Source: CAD feature listing. Evaluate the final solid. Frame: model axes, mm. Face numbers are marked on the shaded views. A direction names the side the tool comes from. Give positions to 0.01 mm unless a question says otherwise; leave off trailing zeros. Loops run counter-clockwise (first coordinate to the right, second up) from the corner with the lowest first, then second, coordinate; pieces in that order, holes last. Notation, with made-up numbers: M -9,14.25 L 13,14.25 A25 ccw 13,35.25 Z; hole C 11,-26 d5. An arc over 180 degrees is marked long. Write item = value, one per line.
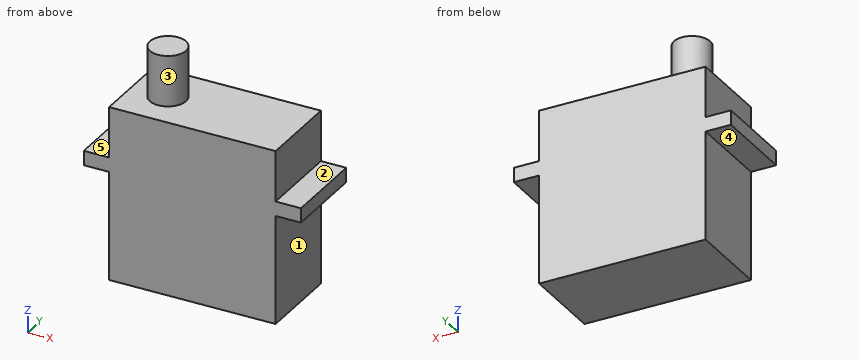
Autodesk Inventor part; units mm, degrees
ref_plane "YZ Plane" through (0, 0, 0) normal (1, 0, 0) x (0, 1, 0)
ref_plane "XZ Plane" through (0, 0, 0) normal (0, 1, 0) x (-1, 0, 0)
ref_plane "XY Plane" through (0, 0, 0) normal (0, 0, 1) x (1, 0, 0)
sketch "Sketch1" plane through (0, 0, 0) normal (0, 0, 1) x (1, 0, 0)
  line L0 (0, 0) -> (23, 0)
  line L1 (23, 0) -> (23, 11.5)
  line L2 (23, 11.5) -> (0, 11.5)
  line L3 (0, 11.5) -> (0, 0)
  dimension "d0" = 23
  dimension "d1" = 11.5
extrude "Extrusion1" add sketch "Sketch1" along normal blind 15
sketch "Sketch2" plane through (0, 0, 15) normal (0, 0, 1) x (1, 0, 0)
  line L0 (23, 11.5) -> (0, 11.5)
  line L1 (0, 11.5) -> (-3.5, 11.5)
  line L2 (-3.5, 11.5) -> (26.5, 11.5)
  line L3 (26.5, 11.5) -> (26.5, 0)
  line L4 (26.5, 0) -> (-3.5, 0)
  line L5 (-3.5, 0) -> (-3.5, 11.5)
  point P0 (0, 0)
  dimension "d4" = 3.5
  dimension "d5" = 30
extrude "Extrusion2" add sketch "Sketch2" along normal blind 2
sketch "Sketch3" plane through (0, 0, 17) normal (0, 0, 1) x (1, 0, 0)
  line L0 (0, 11.5) -> (0, 0)
  line L1 (23, 0) -> (23, 11.5)
  line L2 (0, 11.5) -> (23, 11.5)
  line L3 (23, 11.5) -> (23, 0)
  line L4 (23, 0) -> (0, 0)
  line L5 (0, 0) -> (0, 11.5)
extrude "Extrusion3" add sketch "Sketch3" along normal blind 7
sketch "Sketch4" plane through (0, 0, 24) normal (0, 0, 1) x (1, 0, 0)
  line L0 (0, 11.5) -> (0, 0)
  line L1 (0, 5.75) -> (5, 5.75)
  circle A0 centre (5, 5.75) radius 2.5
  dimension "d10" = 5
  dimension "d11" = 5
extrude "Extrusion4" add sketch "Sketch4" along normal blind 7
properties part number "AilServoRep"
1. First-contact query: pin 1 Ø6 at (y, z) = (7.5, 7) entering from +X; pin 2 Ø1.8 at (x, y) = (-2, 8) entering from +Z; pin 3 Ø2 at (y, z) = (3, 19) entering from -X. Flat tips, straight axial feed; report the tip coordinate or a pass-through.
Derived:
pin_1 = 23
pin_2 = 17
pin_3 = 0
2. Cut plane D-D, the plane y = 5.75. Return the cut outline in (x, z), then the cut area to 3 significant figures.
Derived:
outline = M -3.5,15 L 0,15 L 0,0 L 23,0 L 23,15 L 26.5,15 L 26.5,17 L 23,17 L 23,24 L 7.5,24 L 7.5,31 L 2.5,31 L 2.5,24 L 0,24 L 0,17 L -3.5,17 Z
area = 601 mm²
3. Cut plane B-B, the plane x = 5. Return the cut outline in (y, z).
Derived:
outline = M 0,0 L 11.5,0 L 11.5,24 L 8.25,24 L 8.25,31 L 3.25,31 L 3.25,24 L 0,24 Z
4. Cut plane C-C, the plane z = 12. Return the cut outline in (x, y).
Derived:
outline = M 0,0 L 23,0 L 23,11.5 L 0,11.5 Z
5. Cut plane A-A, the plane y = 9.5. Return the cut outline in (x, z).
Derived:
outline = M -3.5,15 L 0,15 L 0,0 L 23,0 L 23,15 L 26.5,15 L 26.5,17 L 23,17 L 23,24 L 0,24 L 0,17 L -3.5,17 Z
6. Reachability of the marked faces 1, 2, 3, 4 and 5 from +Z, -Z, +X, -X, +Y, -Y: full face, straight path, thin tool, end or side. Return the list, or none.
Derived:
face_1 = -Z, +X, +Y, -Y
face_2 = +Z, +X, +Y, -Y
face_3 = +Z
face_4 = -Z, -X, +Y, -Y
face_5 = +Z, -X, +Y, -Y
7. Material intervals for probe 1 along X at (y, z) = (3.5, 3.5); probe 2 along Z at (x, y) = (2.25, 4.5); probe 3 along Z at (x, y) = (25, 4.75), sorted ascending. Write a range as from..to.
Derived:
probe_1 = 0..23
probe_2 = 0..24
probe_3 = 15..17
